```python
from build123d import *

# Parameters (mm, degrees)
BOSS_EXTRUDE1_DEPTH = 44
CUT_EXTRUDE1_DEPTH  = 44


with BuildPart() as part:
    # Sketch1 → Boss-Extrude1 (new body)
    with BuildSketch(Plane(origin=(0, 0, 0), x_dir=(1, 0, 0), z_dir=(0, 1, 0))):
        Polygon((-9.579875479, -19.511993177), (36.420124521, -19.511993177), (36.420124521, 26.488006823), (34.420124521, 26.488006823), (34.420124521, -17.511993177), (-9.579875479, -17.511993177), align=None)
    extrude(amount=BOSS_EXTRUDE1_DEPTH)

    # Sketch2 → Cut-Extrude1 (cut)
    with BuildSketch(Plane.XY.offset(19.511993177)):
        with BuildLine():
            ThreePointArc((28.420124521, 22), (13.420124521, 37), (-1.579875479, 22))
            Line((-1.579875479, 22), (28.420124521, 22))
        make_face()
        with BuildLine():
            Line((28.420124521, 22), (-1.579875479, 22))
            ThreePointArc((-1.579875479, 22), (13.420124521, 7), (28.420124521, 22))
        make_face()
    extrude(amount=-CUT_EXTRUDE1_DEPTH, mode=Mode.SUBTRACT)


solid = part.part
```
Build history of the part. All positions in model axes, mm. A direction names the side the tool comes from. Coordinates: 2 decimals unless noted, no trailing zeros. Order: outer loops, then holes, each group sorted by start corner. A loop starts at its lowest first (then second) coordinate and runs counter-clockwise, first axis right, second up. Notation, with made-up numbers: (-31.5, 86.5) -> (19.5, 86.5) arc R31 ccw to (19.5, 120.5) -> close; hole circle Ø2 at (5.25, 71.5). An arc over 180 degrees is marked (long way). Answer in a Markdown table with one row per item. Add a question column.
Q1. Drop flat-ended pins along their axis: pin 1 (12 mm diameter, centred on x = 11, y = 31, fed in from +Z); pin 2 (4 mm diameter, centred on y = 27.5, z = -18.5, fed in from -X). Give the stop position or say it passes through.
Q2. Band-saw the part on D-D, the plane y = 35. List the corners of the cut face in (x, z), then the cut area to 3 significant figures.
Q3. Band-saw the part on B-B, the plane x = 22. List the corners of the cut face in (y, z).
Q4. Wall check: line 1 along X through (y, z) = (22, 18.35); line 2 along X through (y, z) = (14.5, -15.5); line 3 along Z through (x, y) = (31.5, 15.5). Give the ranges that are in metal, low to high. Write a range as [from, to].
Q5. Band-saw the part on A-A, the plane y = 22. List the corners of the cut face in (x, z).
Q6. Which spindle directions (+Z, -Z, +X, -X, +Y, -Y) get a long thin tool onto all of the face, cutting with end or side? Do faces 1 (the face through (-2, 22, 17.512)), 2 (the face through (35, 22, -26.488)). Say none if no direction does.
Q7. Mould opens along X. For faces 3 (the face through (-0.436, 27.745, 18.526)), 4 (the face through (35, 44, 7)), 5 (the face through (-9.58, 22, 18)) say: +X half, -X half, draft (parallel to the pull), parting line (faces both ways), or undercut.
Q8. Band-saw the part on C-C, the plane z = -15. List the corners of the cut face in (x, y).
Answers follow:
| question | item | result |
|---|---|---|
| 1 | pin 1 | z = 19.51 |
| 1 | pin 2 | x = 34.42 |
| 2 | outline | (-9.58, 17.51) -> (5.94, 17.51) -> (5.94, 19.51) -> (-9.58, 19.51) -> close; (20.9, 17.51) -> (34.42, 17.51) -> (34.42, -26.49) -> (36.42, -26.49) -> (36.42, 19.51) -> (20.9, 19.51) -> close |
| 2 | area | 150 mm^2 |
| 3 | outline | (0, 17.51) -> (9.7, 17.51) -> (9.7, 19.51) -> (0, 19.51) -> close; (34.3, 17.51) -> (44, 17.51) -> (44, 19.51) -> (34.3, 19.51) -> close |
| 4 | line 1 | [-9.58, -1.58], [28.42, 36.42] |
| 4 | line 2 | [34.42, 36.42] |
| 4 | line 3 | [17.51, 19.51] |
| 5 | outline | (-9.58, 17.51) -> (-1.58, 17.51) -> (-1.58, 19.51) -> (-9.58, 19.51) -> close; (28.42, 17.51) -> (34.42, 17.51) -> (34.42, -26.49) -> (36.42, -26.49) -> (36.42, 19.51) -> (28.42, 19.51) -> close |
| 6 | face 1 | -Z, -X, +Y, -Y |
| 6 | face 2 | -Z, +X, -X, +Y, -Y |
| 7 | face 3 | undercut |
| 7 | face 4 | draft |
| 7 | face 5 | -X half |
| 8 | outline | (34.42, 0) -> (36.42, 0) -> (36.42, 44) -> (34.42, 44) -> close |
